The listing builds one solid part. Answer for the finished solid, in the listing's coordinates (mm). Give positions to 0.01 mm unless a question says otherwise; leave off trailing zeros. Order: outer loops, then holes, each group sorted by start corner. A loop starts at its lowest first (then second) coordinate and runs counter-clockwise, first axis right, second up. Notation, with made-up numbers: (69, 71.5) - (112, 71.5) arc R34 ccw to (112, 109.5) - close; hole circle Ø7 at (60.5, 39.5). An arc over 180 degrees is marked (long way). Write each question's results on one line, items separated by ' | '. Start each with the question number.
1. Section C-C (y = 9.25) is taken. Give the vertices of the cut face in (x, z).
2. Section B-B (z = 0) is taken. Give the vertices of the cut face in (x, y), and give its area (3 significant figures).
3. Section A-A (x = 0) is taken. Give the vertices of the cut face in (y, z), and give its area (3 significant figures).
4. Section D-D (z = -4.5) is taken. Give the vertices of the cut face in (x, y).
5. Determine the mould class of faces 1 (the face through (29, 5, 0)), 2 (the face through (55.645, 2.465, -0.052)), 3 (the face through (1.897, 5, 0)) for opening direction Z: released by +Z, released by -Z, zero draft, split by the parting line, or undercut.
6. Find the intervals of material crossed by L1, parallel to Z at x = 0, y = 3; L2, parallel to X at y = 6.75, z = 0; L3, parallel to Y at x = 36, z = 3.5, in increasing order.
7. Flat-ended cylindrical pins translate along their axes: pin 1 (7.5 mm diameter, centred on x = 39, z = -3.5, fed in from +Y); pin 2 (6 mm diameter, centred on y = 7.5, z = -3.5, fed in from -X); pin 3 (4 mm diameter, centred on x = 7.5, y = 1.5, fed in from +Z). Find the tip coordinate at first contact, or state that the pin passes through.
from build123d import *
from build123d.topology import SkipClean

# Parameters (mm, degrees)
EXTRUDE_1_DEPTH     = 5
SKETCH_2_R          = 7.5
EXTRUDE_2_DEPTH     = 5
CUT_EXTRUDE_1_DEPTH = 58.031822398


with BuildPart() as part:
    # 草图1 → 凸台-拉伸1 (new body)
    with BuildSketch(Plane(origin=(0, 0, 0), x_dir=(1, 0, 0), z_dir=(0, 1, 0))):
        with BuildLine():
            Line((0.705615189, 7.466733369), (53.380319548, 2.488911123))
            ThreePointArc((53.380319548, 2.488911123), (55.645114485, 0), (53.380319548, -2.488911123))
            Line((53.380319548, -2.488911123), (0.705615189, -7.466733369))
            ThreePointArc((0.705615189, -7.466733369), (-7.5, 0), (0.705615189, 7.466733369))
        make_face()
    extrude(amount=EXTRUDE_1_DEPTH)

    # 草图2 → 凸台-拉伸2 (add)
    with SkipClean():  # the faces are left unmerged after this step: merging them gives an invalid solid
        with BuildSketch(Plane(origin=(0, 5, 0), x_dir=(1, 0, 0), z_dir=(0, 1, 0))):
            with Locations(Location((0, 0, 0), (0, 0, 84.601512911))):
                Circle(SKETCH_2_R)
        extrude(amount=EXTRUDE_2_DEPTH)

    # 草图3 → 切除-拉伸1 (cut, through all)
    with SkipClean():  # the faces are left unmerged after this step: merging them gives an invalid solid
        with BuildSketch(Plane(origin=(0, 10, 0), x_dir=(1, 0, 0), z_dir=(0, 1, 0))):
            with BuildLine():
                Line((1.897388784, 1.20930385), (1.897388784, -1.20930385))
                ThreePointArc((1.897388784, -1.20930385), (-2.25, 0), (1.897388784, 1.20930385))
            make_face()
        extrude(amount=-CUT_EXTRUDE_1_DEPTH, mode=Mode.SUBTRACT)


solid = part.part
Reported:
1) outline: circle Ø15 at (0, 0); hole (1.9, -1.21) - (1.9, 1.21) arc R2.25 ccw (long way) to start
2) outline: (-7.5, 0) - (-2.25, 0) - (-2.25, 10) - (-7.5, 10) - close; (1.9, 0) - (55.65, 0) - (55.65, 5) - (7.5, 5) - (7.5, 10) - (1.9, 10) - close | area: 349 mm²
3) outline: (0, -7.5) - (10, -7.5) - (10, -2.25) - (0, -2.25) - close; (0, 2.25) - (10, 2.25) - (10, 7.5) - (0, 7.5) - close | area: 105 mm²
4) outline: (-6, 0) - (32.1, 0) - (32.1, 5) - (6, 5) - (6, 10) - (-6, 10) - close
5) face 1: zero draft | face 2: split by the parting line | face 3: undercut
6) L1: -7.5 to -2.25, 2.25 to 7.5 | L2: -7.5 to -2.25, 1.9 to 7.5 | L3: 0 to 5
7) pin 1: y = 5 | pin 2: x = -7.48 | pin 3: z = 7.01
